```python
from build123d import *

# Parameters (mm, degrees)
SKETCH1_W           = 142.5
SKETCH1_H           = 255
BOSS_EXTRUDE1_DEPTH = 43
SKETCH2_W           = 129.5
SKETCH2_H           = 249
CUT_EXTRUDE1_DEPTH  = 40
BOSS_EXTRUDE2_DEPTH = 79
BOSS_EXTRUDE3_DEPTH = 250


with BuildPart() as part:
    # Sketch1 → Boss-Extrude1 (new body)
    with BuildSketch(Plane(origin=(0, 0, 0), x_dir=(1, 0, 0), z_dir=(0, 1, 0))):
        with Locations((71.25, 127.5)):
            Rectangle(SKETCH1_W, SKETCH1_H)
    extrude(amount=BOSS_EXTRUDE1_DEPTH)

    # Sketch2 → Cut-Extrude1 (cut)
    with BuildSketch(Plane(origin=(0, 43, 0), x_dir=(1, 0, 0), z_dir=(0, 1, 0))):
        with Locations((74.75, 127.5)):
            Rectangle(SKETCH2_W, SKETCH2_H)
    extrude(amount=-CUT_EXTRUDE1_DEPTH, mode=Mode.SUBTRACT)

    # Sketch5 → Boss-Extrude2 (add)
    with BuildSketch(Plane.XY.offset(-3)):
        Polygon((10, 43), (10, 68), (40, 68), (40, 73), (0, 73), (0, 43), align=None)
    extrude(amount=-BOSS_EXTRUDE2_DEPTH)

    # Sketch6 → Boss-Extrude3 (add)
    with BuildSketch(Plane.XY.offset(-3)):
        Polygon((10, 3), (139.5, 42.592123249), (139.5, 3), align=None)
    extrude(amount=-BOSS_EXTRUDE3_DEPTH)


solid = part.part
```
The model under review builds one solid part; all positions refer to its coordinate system, in mm. A direction names the side the tool comes from. Round coordinates to 2 decimals unless told otherwise and drop trailing zeros. Order: outer loops, then holes, each group sorted by start corner. A loop starts at its lowest first (then second) coordinate and runs counter-clockwise, first axis right, second up.
Item 1: Add section A-A, the plane x = 30. State the section outline as (y, z) points, and give its area (3 significant figures).
Working result:
outline: (0, -255) - (43, -255) - (43, -252) - (9.11, -252) - (9.11, -3) - (43, -3) - (43, 0) - (0, 0) - close; (68, -82) - (73, -82) - (73, -3) - (68, -3) - close
area: 2,920 mm2
Item 2: Add section B-B, the plane z = -67. State the section outline as (x, y) points, and give its area (3 significant figures).
Working result:
outline: (0, 0) - (142.5, 0) - (142.5, 43) - (139.5, 43) - (139.5, 42.59) - (10, 3) - (10, 68) - (40, 68) - (40, 73) - (0, 73) - close
area: 3,960 mm2
Item 3: Machinability: for faces 4 (the flat face through (25, 68, -42)), 5 (the flat face through (10.8, 68.2, -3)), 6 (the flat face through (59, 28, -252)), which of the approach directions +Z, -Z, +X, -X, +Y, -Y give a long, thin tool a straight path to every point of the face, cutting with its end or side? Answer none if there is none.
Working result:
face 4: +Z, -Z, +X
face 5: +Z, +X, -X, +Y
face 6: +Y
Item 4: For pin 1 (24 mm diameter, centred on x = 27.5, y = 63.5, fed in from +Z); pin 2 (8 mm diameter, centred on x = 21, z = -224, fed in from +Y); pin 3 (2.5 mm diameter, centred on y = 70, z = -38.5, fed in from +X), all flat-tipped, find the tip position at first contact; note any pin that passes through.
Working result:
pin 1: stops at z = -3
pin 2: stops at y = 7.59
pin 3: stops at x = 40
Item 5: To check wall thickness, follow probe 1 along Z at (x, y) = (92, 36); probe 2 along X at (y, z) = (62, -70); probe 3 along Y at (x, z) = (135, -110.5). State the ranges of each line that lie inside material, in increasing order.
Working result:
probe 1: z = -255 to -252, -3 to 0
probe 2: x = 0 to 10
probe 3: y = 0 to 41.22
Item 6: Add section D-D, the plane x = 79. State the section outline as (y, z) points, and give its area (3 significant figures).
Working result:
outline: (0, -255) - (43, -255) - (43, -252) - (24.1, -252) - (24.1, -3) - (43, -3) - (43, 0) - (0, 0) - close
area: 6,260 mm2
Item 7: Add section C-C, the plane y = 20.5. State the section outline as (x, z) points.
Working result:
outline: (0, -255) - (142.5, -255) - (142.5, 0) - (0, 0) - close; hole (10, -252) - (67.24, -252) - (67.24, -3) - (10, -3) - close
Item 8: Draft analysis for pull direction Z (two halves, no side actions). For faces 1 (the flat face through (0, 29, -97)), 2 (the flat face through (70, 21, 0)), 3 (the flat face through (10, 28, -126)), state which applies: released by +Z, released by -Z, zero draft, split by the parting line, or undercut.
Working result:
face 1: zero draft
face 2: released by +Z
face 3: undercut
